from build123d import *

# Parameters (mm, degrees)
F0_R     = 2.3114
F1_DEPTH = 9.525
F0_W     = 35.56
F0_H     = 8.0197834706
F2_DEPTH = 32.385
F3_R     = 2.3114
F4_DEPTH = 25.4


with BuildPart() as f1:
    # F0 (on Top) → F1 (new body)
    with BuildSketch(Plane.XY):
        Polygon((-10.273542943, 15.6310927123), (-45.833542943, 15.6310927123), (-45.833542943, 13.4908761829), (-45.833542943, -7.2289072877), (-10.273542943, -7.2289072877), align=None)
        with Locations((-40.753542943, -2.1489072877)):
            Circle(F0_R, mode=Mode.SUBTRACT)
        with Locations((-28.053542943, -2.1489072877)):
            Circle(F0_R, mode=Mode.SUBTRACT)
        with Locations((-15.353542943, -2.1489072877)):
            Circle(F0_R, mode=Mode.SUBTRACT)
        with Locations((-40.753542943, 10.5510927123)):
            Circle(F0_R, mode=Mode.SUBTRACT)
        with Locations((-28.053542943, 10.5510927123)):
            Circle(F0_R, mode=Mode.SUBTRACT)
        with Locations((-15.353542943, 10.5510927123)):
            Circle(F0_R, mode=Mode.SUBTRACT)
    extrude(amount=F1_DEPTH)

    # F0 (on Top) → F2 (join)
    with BuildSketch(Plane.XY):
        with Locations((-28.053542943, 19.6409844476)):
            Rectangle(F0_W, F0_H)
    extrude(amount=F2_DEPTH)

    # F3 (on face) → F4 (cut)
    with BuildSketch(Plane.XZ.offset(-15.6310927123)):
        with Locations((-40.753542943, 27.305)):
            Circle(F3_R)
        with Locations((-28.053542943, 27.305)):
            Circle(F3_R)
        with Locations((-15.353542943, 27.305)):
            Circle(F3_R)
        with Locations((-15.353542943, 14.605)):
            Circle(F3_R)
        with Locations((-28.053542943, 14.605)):
            Circle(F3_R)
        with Locations((-40.753542943, 14.605)):
            Circle(F3_R)
    extrude(amount=-F4_DEPTH, mode=Mode.SUBTRACT)


solid = f1.part
Source: CAD feature listing. Evaluate the final solid. Frame: model axes, mm. A direction names the side the tool comes from. Coordinates: 2 decimals unless noted, no trailing zeros. Loops run counter-clockwise (first coordinate to the right, second up) from the corner with the lowest first, then second, coordinate; pieces in that order, holes last. Notation, with made-up numbers: (75, -39.5) -> (127, -39.5) arc R10 ccw to (127, -22.5) -> close; hole circle Ø7 at (-27.75, 45.5). An arc over 180 degrees is marked (long way). Answer in a Markdown table with one row per item. Add a question column.
Q1. Section C-C on y = -1. Return the cut outline in (x, z) (3 decimals).
Q2. Section D-D on z = 3. Return the cut outline in (x, y), and give its area (3 significant figures).
Q3. Section B-B on x = -13.5. Return the cut outline in (y, z) (3 decimals), and give its area (3 significant figures).
Q4. Reachability of faces 4 (the face through (-28, 15.631, 21)), 5 (the face through (-45.834, 11, 9)) from +Z, -Z, +X, -X, +Y, -Y: full face, straight path, thin tool, end or side. Return the list, or none.
Q5. Contact query for flat-ended pins moving along their axis: pin 1 Ø11.5 at (x, y) = (-29.5, 9.5) entering from +Z (3 decimals); pin 2 Ø10 at (x, z) = (-24.5, 20.5) entering from -Y. Output: stop coordinate, or through.
Q6. Section A-A on z = 28. Return the cut outline in (x, y).
Q7. Ray query, line 1 along Z through (x, y) = (-17, 16) (3 decimals); line 2 along Z through (x, y) = (-27, 22) (3 decimals); line 3 along Z through (x, y) = (-18, 1.5) (3 decimals). Return the intervals inside material, ascending.
Q8. Pull-direction query (Y, two-part tool) for faces 1 (the face through (-30.363, 19.585, 27.407)), 2 (the face through (-13.15, -1.45, 4.7)), 3 (the face through (-28, -7.229, 5)); classes: pulls with the +Y half, pulls with the -Y half, needs draft (parallel to the pull), parting line crosses it, or undercut.
Computed values:
| question | item | result |
|---|---|---|
| 1 | outline | (-45.834, 0) -> (-42.759, 0) -> (-42.759, 9.525) -> (-45.834, 9.525) -> close; (-38.748, 0) -> (-30.059, 0) -> (-30.059, 9.525) -> (-38.748, 9.525) -> close; (-26.048, 0) -> (-17.359, 0) -> (-17.359, 9.525) -> (-26.048, 9.525) -> close; (-13.348, 0) -> (-10.274, 0) -> (-10.274, 9.525) -> (-13.348, 9.525) -> close |
| 2 | outline | (-45.83, -7.23) -> (-10.27, -7.23) -> (-10.27, 23.65) -> (-45.83, 23.65) -> close; hole circle Ø4.62 at (-40.75, -2.15); hole circle Ø4.62 at (-40.75, 10.55); hole circle Ø4.62 at (-28.05, -2.15); hole circle Ø4.62 at (-28.05, 10.55); hole circle Ø4.62 at (-15.35, -2.15); hole circle Ø4.62 at (-15.35, 10.55) |
| 2 | area | 997 mm^2 |
| 3 | outline | (-7.229, 0) -> (-3.53, 0) -> (-3.53, 9.525) -> (-7.229, 9.525) -> close; (-0.768, 0) -> (9.17, 0) -> (9.17, 9.525) -> (-0.768, 9.525) -> close; (11.932, 0) -> (23.651, 0) -> (23.651, 13.224) -> (15.631, 13.224) -> (15.631, 9.525) -> (11.932, 9.525) -> close; (15.631, 15.986) -> (23.651, 15.986) -> (23.651, 25.924) -> (15.631, 25.924) -> close; (15.631, 28.686) -> (23.651, 28.686) -> (23.651, 32.385) -> (15.631, 32.385) -> close |
| 3 | area | 381 mm^2 |
| 4 | face 4 | +Z, +X, -X, -Y |
| 4 | face 5 | +Z, -Z, -X, +Y, -Y |
| 5 | pin 1 | stops at z = 9.525 |
| 5 | pin 2 | stops at y = 15.63 |
| 6 | outline | (-45.83, 15.63) -> (-42.96, 15.63) -> (-42.96, 23.65) -> (-45.83, 23.65) -> close; (-38.55, 15.63) -> (-30.26, 15.63) -> (-30.26, 23.65) -> (-38.55, 23.65) -> close; (-25.85, 15.63) -> (-17.56, 15.63) -> (-17.56, 23.65) -> (-25.85, 23.65) -> close; (-13.15, 15.63) -> (-10.27, 15.63) -> (-10.27, 23.65) -> (-13.15, 23.65) -> close |
| 7 | line 1 | z = 0 to 12.983, 16.227 to 25.683, 28.927 to 32.385 |
| 7 | line 2 | z = 0 to 12.548, 16.662 to 25.248, 29.362 to 32.385 |
| 7 | line 3 | z = 0 to 9.525 |
| 8 | face 1 | needs draft |
| 8 | face 2 | undercut |
| 8 | face 3 | pulls with the -Y half |
